The model under review builds one solid part; all positions refer to its coordinate system, in mm. Face numbers are marked on the shaded views. A direction names the side the tool comes from. Coordinates: 2 decimals unless noted, no trailing zeros. Order: outer loops, then holes, each group sorted by start corner. A loop starts at its lowest first (then second) coordinate and runs counter-clockwise, first axis right, second up.
from build123d import *

# Parameters (mm, degrees)
F0_W      = 17
F0_H      = 25
F1_DEPTH  = 2
F0_W_2    = 2
F2_DEPTH  = 45
F3_W      = 2
F3_H      = 7
F4_DEPTH  = 3
F5_R      = 2
F6_R      = 2
F7_R      = 2
F8_R      = 2
F9_R      = 0.99999
F12_DEPTH = 2
F13_DEPTH = 2
F14_W     = 53
F14_H     = 68
F15_DEPTH = 3
F14_W_2   = 57
F14_H_2   = 72
F16_DEPTH = 23
F17_W     = 52.9679324031
F17_H     = 2
F18_DEPTH = 20
F19_DEPTH = 0.7
F21_DEPTH = 5
F22_W     = 87
F22_H     = 65
F23_DEPTH = 13
F25_W     = 83
F25_H     = 10
F26_DEPTH = 11
F24_W     = 10
F24_H     = 83
F27_DEPTH = 45
F28_DEPTH = 45
F29_DEPTH = 45


# Not quite as in the source:
# - a fillet or chamfer is up to 0.001 mm smaller than in the source, because OpenCascade refuses the exact size


with BuildPart() as f1:
    # F0 (on Top) → F1 (new body)
    with BuildSketch(Plane.XY):
        with Locations((22.646613881, -23.1278307736)):
            Rectangle(F0_W, F0_H)
    extrude(amount=F1_DEPTH)

    # F0 (on Top) → F2 (join)
    with BuildSketch(Plane.XY):
        with Locations((32.146613881, -23.1278307736)):
            Rectangle(F0_W_2, F0_H)
    extrude(amount=F2_DEPTH)

    # F3 (on face) → F4 (join)
    with BuildSketch(Plane.XY.offset(45)):
        Polygon((29.146613881, -26.6278307736), (31.146613881, -26.6278307736), (31.146613881, -19.6278307736), (23.146613881, -19.6278307736), (23.146613881, -25.5845747888), (23.146613881, -26.6278307736), align=None)
        with Locations((32.146613881, -23.1278307736)):
            Rectangle(F3_W, F3_H)
    extrude(amount=F4_DEPTH)

    # F5
    f5_edges = [f1.edges().sort_by_distance(p)[0] for p in [
        (23.146614, -23.127831, 48),
    ]]
    fillet(f5_edges, radius=F5_R)

    # F6
    f6_edges = [f1.edges().sort_by_distance(p)[0] for p in [
        (29.146614, -26.627831, 48),
    ]]
    fillet(f6_edges, radius=F6_R)

    # F7
    f7_edges = [f1.edges().sort_by_distance(p)[0] for p in [
        (29.146614, -19.627831, 48),
    ]]
    fillet(f7_edges, radius=F7_R)

    # F8
    f8_edges = [f1.edges().sort_by_distance(p)[0] for p in [
        (33.146614, -23.127831, 48),
    ]]
    fillet(f8_edges, radius=F8_R)

    # F9 (radius 1 in the source; OpenCascade refuses exactly that, so slightly less here)
    f9_edges = [f1.edges().sort_by_distance(p)[0] for p in [
        (23.146614, -23.127831, 45),
    ]]
    fillet(f9_edges, radius=F9_R)

    # F11 (on face) → F12 (join)
    with BuildSketch(Plane.XZ.offset(35.6278307736)):
        Polygon((31.146613881, 2), (31.146613881, 20.3421052632), (14.146613881, 2), align=None)
    extrude(amount=-F12_DEPTH)

    # F10 (on face) → F13 (join)
    with BuildSketch(Plane(origin=(0, -10.6278307736, 0), x_dir=(-1, 0, 0), z_dir=(0, 1, 0))):
        Polygon((-14.146613881, 2), (-31.146613881, 20.3421052632), (-31.146613881, 2), align=None)
    extrude(amount=-F13_DEPTH)


with BuildPart() as f15:
    # F14 (on Top) → F15 (new body)
    with BuildSketch(Plane.XY):
        with Locations((61.8922058344, 0.291702956)):
            Rectangle(F14_W, F14_H)
    extrude(amount=F15_DEPTH)

    # F14 (on Top) → F16 (join)
    with BuildSketch(Plane.XY):
        with Locations((61.8922058344, 0.291702956)):
            Rectangle(F14_W_2, F14_H_2)
        with Locations((61.8922058344, 0.291702956)):
            Rectangle(F14_W, F14_H, mode=Mode.SUBTRACT)
    extrude(amount=F16_DEPTH)

    # F17 (on face) → F18 (cut)
    with BuildSketch(Plane.XY.offset(23)):
        with Locations((61.8761720359, -34.708297044)):
            Rectangle(F17_W, F17_H)
    extrude(amount=-F18_DEPTH, mode=Mode.SUBTRACT)


with BuildPart() as f19:
    # F19 (new): a face of the model
    f19_faces = [f15.part.faces().sort_by_distance(p)[0] for p in [
        (33.3922058344, 0.291702956, 11.5),
    ]]
    extrude(f19_faces, amount=F19_DEPTH)


with BuildPart() as f1_1:
    add(f1.part)

    # F20: union F19, F15
    add(f19.part)
    add(f15.part)

    # F21 (cut): a face of the model
    f21_faces = [f1_1.faces().sort_by_distance(p)[0] for p in [
        (61.5422058344, 35.3690280403, 23),
    ]]
    extrude(f21_faces, amount=-F21_DEPTH, mode=Mode.SUBTRACT)

    # F22 (on face) → F23 (join)
    with BuildSketch(Plane.YZ.offset(90.3922058344)):
        with Locations((7.791702956, 32.5)):
            Rectangle(F22_W, F22_H)
    extrude(amount=F23_DEPTH)

    # F25 (on face) → F26 (cut)
    with BuildSketch(Plane.YZ.offset(103.3922058344)):
        with Locations((7.791702956, 5)):
            Rectangle(F25_W, F25_H)
    extrude(amount=-F26_DEPTH, mode=Mode.SUBTRACT)

    # F24 (on face) → F27 (join)
    with BuildSketch(Plane.XY.offset(65)):
        with Locations((96.8922058344, 7.791702956)):
            Rectangle(F24_W, F24_H)
    extrude(amount=-F27_DEPTH)

    # F24 (on face) → F28 (join)
    with BuildSketch(Plane.XY.offset(65)):
        with Locations((96.8922058344, 7.791702956)):
            Rectangle(F24_W, F24_H)
    extrude(amount=-F28_DEPTH)

    # F24 (on face) → F29 (cut)
    with BuildSketch(Plane.XY.offset(65)):
        with Locations((96.8922058344, 7.791702956)):
            Rectangle(F24_W, F24_H)
    extrude(amount=-F29_DEPTH, mode=Mode.SUBTRACT)


solid = f1_1.part
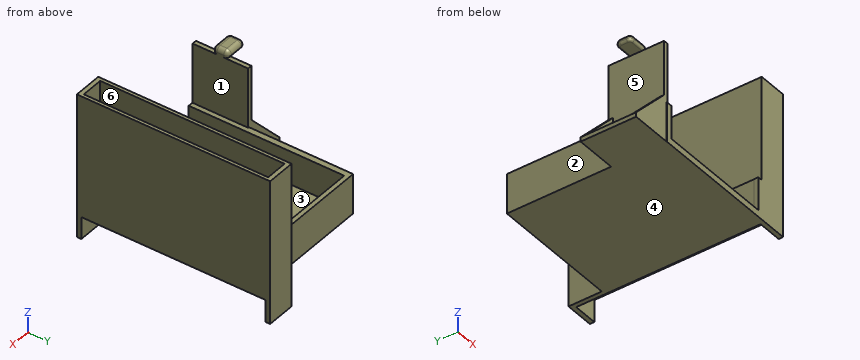
(1) Consider section B-B (x = 95). Give the boundary of the cut face in (y, z).
(2) The part is to be moulded in two halves that separate along X. For the marked faces 4, 5 and 6, say which applies: +X half, -X half, draft (parallel to the pull), parting line (faces both ways), or undercut.
(3) Insertion check: pin 1 Ø7.5 at (y, z) = (-22, 20) entering from -X; pin 2 Ø12 at (y, z) = (26, 12) entering from -X; pin 3 Ø12 at (x, z) = (23.5, 32.5) entering from -Y; pin 4 Ø5 at (y, z) = (15.5, 22) entering from -X. Each pin has a flat end and moves straight along its axis. Give the tip position at first contact, or say it passes through.
(4) Wall thickness on line 1 (X direction, y = -8, z = 21); line 2 (X direction, y = 19, z = 8.5); line 3 (Z direction, x = 62, y = -26): over which ranges is each line inside the solid? List them lowest first.
(5) Tool access review of the marked faces 1, 2 and 3: name each direction out of +Z, -Z, +X, -X, +Y, -Y from which nothing blocks a thin tool from reaching the whole face with its end or side.
(6) Consider section A-A (z = 23.5). Give the boundary of the cut face in (x, y).
Findings:
1. outline: (-35.71, 0) - (-33.71, 0) - (-33.71, 10) - (49.29, 10) - (49.29, 0) - (51.29, 0) - (51.29, 65) - (49.29, 65) - (49.29, 20) - (-33.71, 20) - (-33.71, 65) - (-35.71, 65) - close
2. face 4: draft
2. face 5: -X half
2. face 6: undercut
3. pin 1: stops at x = 31.15
3. pin 2: stops at x = 32.69
3. pin 3: passes through
3. pin 4: stops at x = 90.39
4. line 1: x = 90.39 to 91.89, 101.89 to 103.39
4. line 2: x = 32.69 to 35.39, 88.39 to 92.39
4. line 3: z = 0 to 3
5. face 1: +Z, +Y, -Y
5. face 2: +Z, -Z, -X, +Y
5. face 3: +Z, -Y
6. outline: (31.15, -35.63) - (33.15, -35.63) - (33.15, -10.63) - (31.15, -10.63) - close; (90.39, -35.71) - (103.39, -35.71) - (103.39, 51.29) - (90.39, 51.29) - close; hole (91.89, -33.71) - (101.89, -33.71) - (101.89, 49.29) - (91.89, 49.29) - close
